Geometry: final body of the model. Coordinates: model frame, mm. Give positions to 0.01 mm unless a question says otherwise; leave off trailing zeros. Write each loop counter-clockwise with the first axis right and the second up, starting at its lowest first coordinate (ties: lowest second). Pieces come first, ordered by that corner, then holes.
Q1. Cut plane B-B on y = 0. Return the cut outline in (x, z), plus the area to 3 significant figures.
Q2. Cut plane A-A on x = -56. Return the cut outline in (y, z), plus the area to 3 significant figures.
Q3. Cut plane D-D on y = -18. Return the cut outline in (x, z).
Q4. Pin query (flat end, axial travel): pin 1 (1 mm diameter, centred on y = -5.5, z = 20, fed in from -X); pin 2 (2 mm diameter, centred on y = 35, z = 18, fed in from -X); pin 3 (6 mm diameter, centred on y = -34.5, z = 19.5, fed in from +X). Return the tip coordinate at first contact, or that it passes through.
Q5. Cut plane C-C on z = 6. Return the cut outline in (x, y), plus the area to 3 significant figures.
Q6. Line query: L1, parallel to Y at x = -14, z = 25.25; L2, parallel to Y at x = -20.5, z = 17; L3, parallel to Y at x = 0, z = 16.5. Output: solid intervals per line, ascending.
```python
from build123d import *

# Parameters (mm, degrees)
SZKIC1_R                    = 65
DODANIE_WYCI_GNI_CIE1_DEPTH = 27
SZKIC2_R                    = 6
SZKIC2_R_2                  = 41
WYTNIJ_WYCI_GNI_CIE1_DEPTH  = 35


with BuildPart() as part:
    # Szkic1 → Dodanie-wyciągnięcie1 (new body)
    with BuildSketch(Plane.XY):
        Circle(SZKIC1_R)
    extrude(amount=DODANIE_WYCI_GNI_CIE1_DEPTH)

    # Szkic2 → Wytnij-wyciągnięcie1 (cut)
    with BuildSketch(Plane.XY.offset(27)):
        with Locations((-56, 0)):
            Circle(SZKIC2_R)
        with Locations((-17.304951685, 53.259164913)):
            Circle(SZKIC2_R)
        with Locations((45.304951685, 32.915974128)):
            Circle(SZKIC2_R)
        with Locations((45.304951685, -32.915974128)):
            Circle(SZKIC2_R)
        with Locations((-17.304951685, -53.259164913)):
            Circle(SZKIC2_R)
        Circle(SZKIC2_R_2)
    extrude(amount=-WYTNIJ_WYCI_GNI_CIE1_DEPTH, mode=Mode.SUBTRACT)


solid = part.part
```
Data:
1. outline: (-65, 0) - (-62, 0) - (-62, 27) - (-65, 27) - close; (-50, 0) - (-41, 0) - (-41, 27) - (-50, 27) - close; (41, 0) - (65, 0) - (65, 27) - (41, 27) - close
1. area: 972 mm2
2. outline: (-33, 0) - (-6, 0) - (-6, 27) - (-33, 27) - close; (6, 0) - (33, 0) - (33, 27) - (6, 27) - close
2. area: 1,460 mm2
3. outline: (-62.46, 0) - (-36.84, 0) - (-36.84, 27) - (-62.46, 27) - close; (36.84, 0) - (62.46, 0) - (62.46, 27) - (36.84, 27) - close
4. pin 1: stops at x = -64.81
4. pin 2: stops at x = -55.4
4. pin 3: stops at x = 56.86
5. outline: circle Ø130 at (0, 0); hole circle Ø12 at (-56, 0); hole circle Ø82 at (0, 0); hole circle Ø12 at (-17.3, -53.26); hole circle Ø12 at (-17.3, 53.26); hole circle Ø12 at (45.3, -32.92); hole circle Ø12 at (45.3, 32.92)
5. area: 7,430 mm2
6. L1: y = -63.47 to -58.27, -48.25 to -38.54, 38.54 to 48.25, 58.27 to 63.47
6. L2: y = -61.68 to -58.34, -48.18 to -35.51, 35.51 to 48.18, 58.34 to 61.68
6. L3: y = -65 to -41, 41 to 65
